Can you work these out from the model? Positions are in its coordinate system, mm. Coordinates: 2 decimals unless noted, no trailing zeros. Order: outer loops, then holes, each group sorted by start corner. A loop starts at its lowest first (then second) coordinate and runs counter-clockwise, first axis right, second up. Notation, with made-up numbers: M 56,63.25 L 74,63.25 A36 ccw 74,101.25 Z; hole C -12,37.25 d1. An arc over 180 degrees is marked long. Answer as CSV lines item,"result". Start each with the question number.
1. I need wall thicknesses on line 1 along Y through (x, z) = (0, 0); line 2 along Y through (x, z) = (-1.25, 0.2); line 3 along X through (y, z) = (-0.5, 0.1). Which ranges of each line are inside material? Lowest first, please. Write a range as from..to.
2. If we section it at A-A (x = 0): List the corners of the cut face in (y, z) for me (3 decimals), plus the area to 3 significant figures.
3. Will this pin go through, and if not, where does the flat tip stop? pin 1 (4 mm diameter, centred on x = 0, y = 0, fed in from -Z) (3 decimals).
4. If we section it at C-C (z = 0.05): List the corners of the cut face in (x, y) for me, plus the area to 3 significant figures.
5. If we mould it in two halves opening along Y, with no side actions, what happens to faces 1 (the face through (-2, -1, 0.275)), 2 (the face through (-1.27, -0.97, -0.04))? For each: released by +Y, released by -Y, zero draft, split by the parting line, or undercut.
```python
from build123d import *

# Parameters (mm, degrees)
SKETCH3_R                = 3.5
SKETCH3_R_2              = 1.6
BOSS_EXTRUDE1_DEPTH      = 0.275
BOSS_EXTRUDE1_DEPTH_BACK = 0.275
FILLET1_R                = 0.14
FILLET2_R                = 0.07


with BuildPart() as part:
    # Sketch3 → Boss-Extrude1 (new body, two sides)
    with BuildSketch(Plane.XY) as boss_extrude1_sk:
        Circle(SKETCH3_R)
        Circle(SKETCH3_R_2, mode=Mode.SUBTRACT)
    extrude(amount=BOSS_EXTRUDE1_DEPTH)
    extrude(boss_extrude1_sk.sketch, amount=-BOSS_EXTRUDE1_DEPTH_BACK)

    # Fillet1
    fillet1_edges = [part.edges().sort_by_distance(p)[0] for p in [
        (-3.5, 0, -0.275),
        (-3.5, 0, 0.275),
    ]]
    fillet(fillet1_edges, radius=FILLET1_R)

    # Fillet2
    fillet2_edges = [part.edges().sort_by_distance(p)[0] for p in [
        (-1.6, 0, 0.275),
    ]]
    fillet(fillet2_edges, radius=FILLET2_R)


solid = part.part
```
Solved:
1,line 1,"-3.5..-1.6, 1.6..3.5"
1,line 2,"-3.25..-1, 1..3.25"
1,line 3,"-3.46..-1.52, 1.52..3.46"
2,outline,"M -3.5,-0.135 A0.14 ccw -3.36,-0.275 L -1.6,-0.275 L -1.6,0.205 A0.07 ccw -1.67,0.275 L -3.36,0.275 A0.14 ccw -3.5,0.135 Z; M 1.6,-0.275 L 3.36,-0.275 A0.14 ccw 3.5,-0.135 L 3.5,0.135 A0.14 ccw 3.36,0.275 L 1.67,0.275 A0.07 ccw 1.6,0.205 Z"
2,area,"2.07 mm²"
3,pin 1,"z = -0.275"
4,outline,"C 0,0 d7; hole C 0,0 d3.2"
4,area,"30.4 mm²"
5,face 1,"zero draft"
5,face 2,"undercut"
